from build123d import *

# Parameters (mm, degrees)
EXTRUDE_7_DEPTH       = 7
CUT_EXTRUDE_START     = 3
CUT_EXTRUDE_3_2_DEPTH = 4
M3_M4_5V_START        = 3
SKETCH_3_W            = 6
SKETCH_3_H            = 58
M3_M4_5V_DEPTH        = 4
M2_M1_START           = 3
SKETCH_4_W            = 6
SKETCH_4_H            = 45
M2_M1_DEPTH           = 4
SKETCH_5_W            = 56
SKETCH_5_H            = 6
CUT_EXTRUDE_M3_DEPTH  = 4
DC_START              = 3
SKETCH_6_W            = 49
SKETCH_6_H            = 6
DC_DEPTH              = 4
EXTRUDE_START         = 3
SKETCH_7_R            = 3
EXTRUDE_5_DEPTH       = 5
SKETCH_8_R            = 1.8
PCB_0_3_DEPTH         = 8


with BuildPart() as part:
    # 草图1 → 底托基础_总边高7 (new body)
    with BuildSketch(Plane.XY):
        with BuildLine():
            Line((-36, -39), (36, -39))
            ThreePointArc((36, -39), (38.121320344, -38.121320344), (39, -36))
            Line((39, -36), (39, 36))
            ThreePointArc((39, 36), (38.121320344, 38.121320344), (36, 39))
            Line((36, 39), (-36, 39))
            ThreePointArc((-36, 39), (-38.121320344, 38.121320344), (-39, 36))
            Line((-39, 36), (-39, -36))
            ThreePointArc((-39, -36), (-38.121320344, -38.121320344), (-36, -39))
        make_face()
    extrude(amount=EXTRUDE_7_DEPTH)

    # 草图2 → 底腔_实体绝缘底厚3_侧壁2 (cut)
    with BuildSketch(Plane.XY.offset(CUT_EXTRUDE_START)):
        with BuildLine():
            Line((-36, -37), (36, -37))
            ThreePointArc((36, -37), (36.707106781, -36.707106781), (37, -36))
            Line((37, -36), (37, 36))
            ThreePointArc((37, 36), (36.707106781, 36.707106781), (36, 37))
            Line((36, 37), (-36, 37))
            ThreePointArc((-36, 37), (-36.707106781, 36.707106781), (-37, 36))
            Line((-37, 36), (-37, -36))
            ThreePointArc((-37, -36), (-36.707106781, -36.707106781), (-36, -37))
        make_face()
    extrude(amount=CUT_EXTRUDE_3_2_DEPTH, mode=Mode.SUBTRACT)

    # 草图3 → 左侧M3_M4编码器及5V接口开口_不切穿绝缘底板 (cut)
    with BuildSketch(Plane.XY.offset(M3_M4_5V_START)):
        with Locations((-39, 4)):
            Rectangle(SKETCH_3_W, SKETCH_3_H)
    extrude(amount=M3_M4_5V_DEPTH, mode=Mode.SUBTRACT)

    # 草图4 → 右侧M2_M1及电机接口开口_不切穿绝缘底板 (cut)
    with BuildSketch(Plane.XY.offset(M2_M1_START)):
        with Locations((39, 10.5)):
            Rectangle(SKETCH_4_W, SKETCH_4_H)
    extrude(amount=M2_M1_DEPTH, mode=Mode.SUBTRACT)

    # 草图5 → 上侧控制与编码器及M3接口开口_不切穿绝缘底板 (cut)
    with BuildSketch(Plane.XY.offset(CUT_EXTRUDE_START)):
        with Locations((0, 39)):
            Rectangle(SKETCH_5_W, SKETCH_5_H)
    extrude(amount=CUT_EXTRUDE_M3_DEPTH, mode=Mode.SUBTRACT)

    # 草图6 → 下侧凤凰端子_DC_电源开关共用开口_不切穿绝缘底板 (cut)
    with BuildSketch(Plane.XY.offset(DC_START)):
        with Locations((-4.5, -39)):
            Rectangle(SKETCH_6_W, SKETCH_6_H)
    extrude(amount=DC_DEPTH, mode=Mode.SUBTRACT)

    # 草图7 → 四根绝缘支柱_板背净距5 (add)
    with BuildSketch(Plane.XY.offset(EXTRUDE_START)):
        with Locations((-18.5, -18.5)):
            Circle(SKETCH_7_R)
        with Locations((-18.5, 18.5)):
            Circle(SKETCH_7_R)
        with Locations((18.5, -18.5)):
            Circle(SKETCH_7_R)
        with Locations((18.5, 18.5)):
            Circle(SKETCH_7_R)
    extrude(amount=EXTRUDE_5_DEPTH)

    # 草图8 → PCB与底部对齐通孔_单边0.3 (cut)
    with BuildSketch(Plane.XY):
        with Locations((-18.5, -18.5)):
            Circle(SKETCH_8_R)
        with Locations((-18.5, 18.5)):
            Circle(SKETCH_8_R)
        with Locations((18.5, -18.5)):
            Circle(SKETCH_8_R)
        with Locations((18.5, 18.5)):
            Circle(SKETCH_8_R)
    extrude(amount=PCB_0_3_DEPTH, mode=Mode.SUBTRACT)


solid = part.part
Model file for the job. Use its own axes, mm. A direction names the side the tool comes from. Round coordinates to 2 decimals unless told otherwise and drop trailing zeros. Loops run counter-clockwise (first coordinate to the right, second up) from the corner with the lowest first, then second, coordinate; pieces in that order, holes last.
1. Drop flat-ended pins along their axis: P1, Ø2, axis at x = 38, z = 5.5, coming from the +Y side; P2, Ø1, axis at x = -22.5, y = 0.5, coming from the +Z side; P3, Ø1, axis at x = -38, z = 5.5, coming from the -Y side; P4, Ø2, axis at x = 18.5, y = 18.5, coming from the +Z side. Give the stop position or say it passes through.
Check values:
P1: stops at y = 38.83
P2: stops at z = 3
P3: stops at y = -38.6
P4: passes through
2. Tool access for faces 1 (the cylindrical face through (-38.1, 38.14, 3.45)), 2 (the flat face through (-29, -38, 5)), 3 (the flat face through (32, 37, 5)): list every direction of +Z, -Z, +X, -X, +Y, -Y with a clear straight run to the whole face (end or side of a thin tool).
Check values:
face 1: +Z, -Z, -X, +Y
face 2: +Z, -Y
face 3: +Z
3. Wall check: probe 1 along Y at (x, z) = (18.5, 6); probe 2 along Y at (x, z) = (-18.5, 1.5); probe 3 along Z at (x, y) = (-27, 33). Give the ranges that are in metal, low to high.
Check values:
probe 1: y = -21.5 to -20.3, -16.7 to -15.5, 15.5 to 16.7, 20.3 to 21.5
probe 2: y = -39 to -20.3, -16.7 to 16.7, 20.3 to 39
probe 3: z = 0 to 3
4. Mould opens along X. For faces 4 (the cylindrical face through (16.1, 16.7, 5.5)), 5 (the cylindrical face through (-20.9, 16.7, 5.5)), 6 (the flat face through (1, 39, 2)), 7 (the cylindrical face through (-38.14, -38.1, 3.45)) say: +X half, -X half, draft (parallel to the pull), parting line (faces both ways), or undercut.
Check values:
face 4: undercut
face 5: undercut
face 6: draft
face 7: -X half
5. Band-saw the part on C-C, the plane z = 5.5. Count the separate pieces of the cut face and the enclosed holes in it, and give its area (3 significant figures).
Check values:
separate pieces: 8
enclosed holes: 4
area: 258 mm2
6. Band-saw the part on A-A, the plane y = 18.5. List the corners of the cut face in (x, z), and give its area (3 significant figures).
Check values:
outline: (-39, 0) - (-20.3, 0) - (-20.3, 8) - (-21.5, 8) - (-21.5, 3) - (-39, 3) - close; (-16.7, 0) - (16.7, 0) - (16.7, 8) - (15.5, 8) - (15.5, 3) - (-15.5, 3) - (-15.5, 8) - (-16.7, 8) - close; (20.3, 0) - (39, 0) - (39, 3) - (21.5, 3) - (21.5, 8) - (20.3, 8) - close
area: 236 mm2
7. Band-saw the part on D-D, the plane x = 25.5. List the corners of the cut face in (y, z).
Check values:
outline: (-39, 0) - (39, 0) - (39, 3) - (-37, 3) - (-37, 7) - (-39, 7) - close
